Input: part model. Units: mm. Frame: model coordinates. A direction names the side the tool comes from. Give positions to 0.01 mm unless a question says otherwise; leave off trailing zeros. Write each loop counter-clockwise with the first axis right and the second up, starting at its lowest first coordinate (ties: lowest second). Pieces come first, ordered by that corner, then holes. Notation, with made-up numbers: (16, 66) - (46, 66) arc R18 ccw to (46, 73) - close; hole circle Ø1 at (47.25, 83.5). An arc over 180 degrees is marked (long way). Use a Markdown table: item, result. Add a question column.
1. Section query B-B, the plane y = 181.5. Return loops of the section in (x, z), plus the area to 3 significant figures.
2. Section query A-A, the plane x = -162. Return loops of the section in (y, z) (3 decimals).
3. Pin query (flat end, axial travel): pin 1 (12.5 mm diameter, centred on x = 312.5, z = 301.5, fed in from -Y) (3 decimals). Return the tip coordinate at first contact, or that it passes through.
4. Section query D-D, the plane y = -129.5. Return loops of the section in (x, z), plus the area to 3 significant figures.
5. Material intervals for probe 1 along Y at (x, z) = (8.5, 527) (3 decimals); probe 2 along X at (y, z) = (190, 116.5), sorted ascending.
6. Section query C-C, the plane z = 431.5. Return loops of the section in (x, y) (3 decimals), plus the area to 3 significant figures.
7. Mould query, pull axis X, two halves, no side actions, for faces 1 (the flat face through (-323.85, 180, 322)), 2 (the flat face through (-298.45, 182, 257)), 3 (the flat face through (73, 219.075, 50)). Classes: released by +X, released by -X, zero draft, split by the parting line, or undercut.
8. Set-up query: faces 4 (the flat face through (-4, -193.675, 25)), 5 (the flat face through (4, 207, 508)), 6 (the flat face through (-311, 168.275, 276)), 7 (the flat face through (298.45, 182, 257)), 8 (the flat face through (-26, -194, 0)). Return all of +Z, -Z, +X, -X, +Y, -Y with unobstructed straight access to the full face (end or side cutting, diameter ignored); none if empty.
```python
from build123d import *

# Parameters (mm, degrees)
F0_W      = 647.7
F0_H      = 438.15
F0_W_2    = 596.9
F0_H_2    = 387.35
F1_DEPTH  = 50.8
F3_DEPTH  = 508
F4_W      = 25.4
F4_H      = 50.8
F5_DEPTH  = 374.65
F6_W      = 25.4
F6_H      = 50.8
F7_DEPTH  = 387.35
F8_W      = 25.4
F8_H      = 50.8
F9_DEPTH  = 622.3
F10_W     = 25.4
F10_H     = 50.8
F11_DEPTH = 622.3


with BuildPart() as f1:
    # F0 (on Top) → F1 (new body)
    with BuildSketch(Plane.XY):
        Rectangle(F0_W, F0_H)
        Rectangle(F0_W_2, F0_H_2, mode=Mode.SUBTRACT)
    extrude(amount=F1_DEPTH)

    # F2 (on face) → F3 (join)
    with BuildSketch(Plane.XY.offset(50.8)):
        Polygon((-298.45, 219.075), (-323.85, 219.075), (-323.85, 168.275), (-298.45, 168.275), (-298.45, 193.675), align=None)
        Polygon((323.85, 219.075), (298.45, 219.075), (298.45, 193.675), (298.45, 168.275), (323.85, 168.275), align=None)
    extrude(amount=F3_DEPTH)

    # F4 (on face) → F5 (join)
    with BuildSketch(Plane.XZ.offset(-168.275)):
        with Locations((-311.15, 533.4)):
            Rectangle(F4_W, F4_H)
    extrude(amount=F5_DEPTH)

    # F6 (on face) → F7 (join)
    with BuildSketch(Plane.XZ.offset(-168.275)):
        with Locations((311.15, 533.4)):
            Rectangle(F6_W, F6_H)
    extrude(amount=F7_DEPTH)

    # F8 (on face) → F9 (join)
    with BuildSketch(Plane(origin=(298.45, 0, 0), x_dir=(0, -1, 0), z_dir=(-1, 0, 0))):
        with Locations((206.375, 533.4)):
            Rectangle(F8_W, F8_H)
    extrude(amount=F9_DEPTH)

    # F10 (on face) → F11 (join)
    with BuildSketch(Plane(origin=(298.45, 0, 0), x_dir=(0, -1, 0), z_dir=(-1, 0, 0))):
        with Locations((-206.375, 533.4)):
            Rectangle(F10_W, F10_H)
    extrude(amount=F11_DEPTH)


solid = f1.part
```
Result sheet:
| question | item | result |
|---|---|---|
| 1 | outline | (-323.85, 0) - (-298.45, 0) - (-298.45, 558.8) - (-323.85, 558.8) - close; (298.45, 0) - (323.85, 0) - (323.85, 558.8) - (298.45, 558.8) - close |
| 1 | area | 28,400 mm² |
| 2 | outline | (-219.075, 0) - (-193.675, 0) - (-193.675, 50.8) - (-219.075, 50.8) - close; (-219.075, 508) - (-193.675, 508) - (-193.675, 558.8) - (-219.075, 558.8) - close; (193.675, 0) - (219.075, 0) - (219.075, 50.8) - (193.675, 50.8) - close; (193.675, 508) - (219.075, 508) - (219.075, 558.8) - (193.675, 558.8) - close |
| 3 | pin 1 | stops at y = 168.275 |
| 4 | outline | (-323.85, 0) - (-298.45, 0) - (-298.45, 50.8) - (-323.85, 50.8) - close; (-323.85, 508) - (-298.45, 508) - (-298.45, 558.8) - (-323.85, 558.8) - close; (298.45, 0) - (323.85, 0) - (323.85, 50.8) - (298.45, 50.8) - close; (298.45, 508) - (323.85, 508) - (323.85, 558.8) - (298.45, 558.8) - close |
| 4 | area | 5,160 mm² |
| 5 | probe 1 | y = -219.075 to -193.675, 193.675 to 219.075 |
| 5 | probe 2 | x = -323.85 to -298.45, 298.45 to 323.85 |
| 6 | outline | (-323.85, 168.275) - (-298.45, 168.275) - (-298.45, 219.075) - (-323.85, 219.075) - close; (298.45, 168.275) - (323.85, 168.275) - (323.85, 219.075) - (298.45, 219.075) - close |
| 6 | area | 2,580 mm² |
| 7 | face 1 | released by -X |
| 7 | face 2 | undercut |
| 7 | face 3 | zero draft |
| 8 | face 4 | +Z, -Z |
| 8 | face 5 | +Y, -Y |
| 8 | face 6 | +X, -X, -Y |
| 8 | face 7 | none |
| 8 | face 8 | -Z, +X, -X, +Y, -Y |
